```python
from build123d import *

# Parameters (mm, degrees)
SKETCH1_W           = 82.8
SKETCH1_H           = 57.7
BOSS_EXTRUDE1_DEPTH = 21.2
SKETCH2_R           = 1.5
CUT_EXTRUDE1_DEPTH  = 22
CUT_EXTRUDE2_DEPTH  = 20
FILLET3_R           = 4
BOSS_EXTRUDE3_START = 1
BOSS_EXTRUDE3_DEPTH = 1
CUT_EXTRUDE6_DEPTH  = 126.949440358
SKETCH8_R           = 3.8
CUT_EXTRUDE7_DEPTH  = 91.96532852
CUT_EXTRUDE8_DEPTH  = 10


with BuildPart() as part:
    # Sketch1 → Boss-Extrude1 (new body)
    with BuildSketch(Plane(origin=(0, 0, 0), x_dir=(1, 0, 0), z_dir=(0, 1, 0))):
        with Locations((-68.529666271, 2.285365627)):
            Rectangle(SKETCH1_W, SKETCH1_H)
    extrude(amount=BOSS_EXTRUDE1_DEPTH)

    # Sketch2 → Cut-Extrude1 (cut)
    with BuildSketch(Plane.XZ):
        with Locations(Location((-105.929666271, 22.574078856, 0), (0, 0, 270))):
            Circle(SKETCH2_R)
        with Locations(Location((-31.129666271, 22.574078856, 0), (0, 0, 270))):
            Circle(SKETCH2_R)
        with Locations(Location((-105.929666271, -27.14481011, 0), (0, 0, 270))):
            Circle(SKETCH2_R)
        with Locations(Location((-31.129666271, -27.14481011, 0), (0, 0, 270))):
            Circle(SKETCH2_R)
    extrude(amount=-CUT_EXTRUDE1_DEPTH, mode=Mode.SUBTRACT)

    # Sketch3 → Cut-Extrude2 (cut)
    with BuildSketch(Plane.XZ):
        with BuildLine():
            Line((-101.969305307, 23.064634373), (-35.090027235, 23.064634373))
            ThreePointArc((-35.090027235, 23.064634373), (-33.948648913, 19.745651731), (-30.629666271, 18.604273409))
            Line((-30.629666271, 18.604273409), (-30.629666271, -23.175004663))
            ThreePointArc((-30.629666271, -23.175004663), (-33.948648913, -24.316382985), (-35.090027235, -27.635365627))
            Line((-35.090027235, -27.635365627), (-101.969305307, -27.635365627))
            ThreePointArc((-101.969305307, -27.635365627), (-103.110683629, -24.316382985), (-106.429666271, -23.175004663))
            Line((-106.429666271, -23.175004663), (-106.429666271, 18.607164142))
            ThreePointArc((-106.429666271, 18.607164142), (-103.111962249, 19.747670443), (-101.969305307, 23.064634373))
        make_face()
    extrude(amount=-CUT_EXTRUDE2_DEPTH, mode=Mode.SUBTRACT)

    # Fillet3
    fillet3_edges = [part.edges().sort_by_distance(p)[0] for p in [
        (-27.129666271, 10.6, 26.564634373),
        (-109.929666271, 10.6, 26.564634373),
        (-109.929666271, 10.6, -31.135365627),
        (-27.129666271, 10.6, -31.135365627),
    ]]
    fillet(fillet3_edges, radius=FILLET3_R)

    # Sketch3_8 → Boss-Extrude3 (add)
    with BuildSketch(Plane.XZ.offset(BOSS_EXTRUDE3_START)):
        with BuildLine():
            Line((-103.334287863, 24.064634373), (-33.723727934, 24.064634373))
            ThreePointArc((-33.723727934, 24.064634373), (-33.241542132, 20.452758513), (-29.629666271, 19.97057271))
            Line((-29.629666271, 19.97057271), (-29.629666271, -24.541303964))
            ThreePointArc((-29.629666271, -24.541303964), (-33.241542132, -25.023489766), (-33.723727934, -28.635365627))
            Line((-33.723727934, -28.635365627), (-103.335604608, -28.635365627))
            ThreePointArc((-103.335604608, -28.635365627), (-103.817790411, -25.023489766), (-107.429666271, -24.541303964))
            Line((-107.429666271, -24.541303964), (-107.429666271, 19.973301106))
            ThreePointArc((-107.429666271, 19.973301106), (-103.819200468, 20.454646008), (-103.334287863, 24.064634373))
        make_face()
        with BuildLine():
            Line((-101.969305307, 23.064634373), (-35.090027235, 23.064634373))
            ThreePointArc((-35.090027235, 23.064634373), (-33.948648913, 19.745651731), (-30.629666271, 18.604273409))
            Line((-30.629666271, 18.604273409), (-30.629666271, -23.175004663))
            ThreePointArc((-30.629666271, -23.175004663), (-33.948648913, -24.316382985), (-35.090027235, -27.635365627))
            Line((-35.090027235, -27.635365627), (-101.969305307, -27.635365627))
            ThreePointArc((-101.969305307, -27.635365627), (-103.110683629, -24.316382985), (-106.429666271, -23.175004663))
            Line((-106.429666271, -23.175004663), (-106.429666271, 18.607164142))
            ThreePointArc((-106.429666271, 18.607164142), (-103.111962249, 19.747670443), (-101.969305307, 23.064634373))
        make_face(mode=Mode.SUBTRACT)
    extrude(amount=-BOSS_EXTRUDE3_DEPTH)

    # Sketch7 → Cut-Extrude6 (cut, through all)
    with BuildSketch(Plane(origin=(0, 0, -31.135365627), x_dir=(-1, 0, 0), z_dir=(0, 0, -1))):
        with BuildLine():
            Line((97.929666271, 10), (60.929666271, 10))
            ThreePointArc((60.929666271, 10), (59.929666271, 9), (60.929666271, 8))
            Line((60.929666271, 8), (97.929666271, 8))
            ThreePointArc((97.929666271, 8), (98.929666271, 9), (97.929666271, 10))
        make_face()
        with BuildLine():
            Line((97.929666271, 5), (60.929666271, 5))
            ThreePointArc((60.929666271, 5), (59.929666271, 4), (60.929666271, 3))
            Line((60.929666271, 3), (97.929666271, 3))
            ThreePointArc((97.929666271, 3), (98.929666271, 4), (97.929666271, 5))
        make_face()
    extrude(amount=-CUT_EXTRUDE6_DEPTH, mode=Mode.SUBTRACT)

    # Sketch8 → Cut-Extrude7 (cut, through all)
    with BuildSketch(Plane.ZY.offset(109.929666271)):
        with Locations((14.564634373, 9.2)):
            Circle(SKETCH8_R)
    extrude(amount=-CUT_EXTRUDE7_DEPTH, mode=Mode.SUBTRACT)

    # Sketch10 → Cut-Extrude8 (cut)
    with BuildSketch(Plane.XY.offset(26.564634373)):
        with BuildLine():
            Line((-43.129666271, 15), (-45.129666271, 15))
            ThreePointArc((-45.129666271, 15), (-47.129666271, 17), (-45.129666271, 19))
            Line((-45.129666271, 19), (-43.129666271, 19))
            ThreePointArc((-43.129666271, 19), (-41.129666271, 17), (-43.129666271, 15))
        make_face()
        with BuildLine():
            Line((-54.879666271, 15), (-56.879666271, 15))
            ThreePointArc((-56.879666271, 15), (-58.879666271, 17), (-56.879666271, 19))
            Line((-56.879666271, 19), (-54.879666271, 19))
            ThreePointArc((-54.879666271, 19), (-52.879666271, 17), (-54.879666271, 15))
        make_face()
        with BuildLine():
            Line((-66.629666271, 15), (-68.629666271, 15))
            ThreePointArc((-68.629666271, 15), (-70.629666271, 17), (-68.629666271, 19))
            Line((-68.629666271, 19), (-66.629666271, 19))
            ThreePointArc((-66.629666271, 19), (-64.629666271, 17), (-66.629666271, 15))
        make_face()
        with BuildLine():
            Line((-78.379666271, 15), (-80.379666271, 15))
            ThreePointArc((-80.379666271, 15), (-82.379666271, 17), (-80.379666271, 19))
            Line((-80.379666271, 19), (-78.379666271, 19))
            ThreePointArc((-78.379666271, 19), (-76.379666271, 17), (-78.379666271, 15))
        make_face()
    extrude(amount=-CUT_EXTRUDE8_DEPTH, mode=Mode.SUBTRACT)


solid = part.part
```
Can you work these out from the model? Positions are in its coordinate system, mm. A direction names the side the tool comes from. Round coordinates to 2 decimals unless told otherwise and drop trailing zeros. Loops run counter-clockwise (first coordinate to the right, second up) from the corner with the lowest first, then second, coordinate; pieces in that order, holes last.
Item 1: If we mould it in two halves opening along Z, with no side actions, what happens to faces 1 (the cylindrical face through (-33.91, 9.35, -24.28)), 2 (the cylindrical face through (-98.93, 3.98, 24.79)), 3 (the cylindrical face through (-28.33, 10.75, -29.99))? For each: +Z half, -Z half, draft (parallel to the pull), parting line (faces both ways), or undercut.
Item 2: Suppose I cut it at C-C, the plane y = 11.5. Write out the boundary of the cut face in (x, z) (3 decimals).
Item 3: Suppose I cut it at A-A, the plane y = 4. Write out the boundary of the cut face in (x, z) (3 decimals).
Item 4: Will these pins go through, and if not, where does the flat tip stop? pin 1 Ø3 at (x, z) = (-86.5, -29) entering from -Y; pin 2 Ø0.5 at (y, z) = (-0.5, 7.5) entering from -X; pin 3 Ø10 at (x, z) = (-77, 5) entering from -Y; pin 4 Ø1.8 at (x, z) = (-76, 25) entering from -Y.
Item 5: Please list where these lines run through material, in increasing order: L1, parallel to Y at x = -81.5, z = -28; L2, parallel to X at y = 17, z = 13.5; L3, parallel to Z at x = -105, y = 16.
Item 6: Suppose I cut it at D-D, the plane y = 17. State how many separate pieces and enclosed holes the cut face has, then the cut area to 3 significant figures.
Item 7: Suppose I cut it at B-B, the plane z = -11.5. Write out the boundary of the cut face in (x, y).
Item 8: Which directions (+Z, -Z, +X, -X, +Y, -Y) give clear straight access to the entire face, cutting with the end or side of a thin tool? Please do faces 4 (the cylindrical face through (-58.88, 16.96, 24.84)), 5 (the flat face through (-68, 12, -27.635)), 6 (the flat face through (-69, 21.2, -3)), 7 (the cylindrical face through (-28.904, 6.888, 11.549)), 8 (the flat face through (-79, 3, -29)).
Reported:
1. face 1: undercut
1. face 2: draft
1. face 3: -Z half
2. outline: (-109.93, -27.135) arc R4 ccw to (-105.93, -31.135) - (-31.13, -31.135) arc R4 ccw to (-27.13, -27.135) - (-27.13, 11.54) - (-30.63, 11.54) - (-30.63, -23.175) arc R4 ccw to (-35.09, -27.635) - (-101.969, -27.635) arc R4 ccw to (-106.43, -23.175) - (-106.43, 11.54) - (-109.93, 11.54) - close; (-109.93, 17.59) - (-106.43, 17.59) - (-106.43, 18.607) arc R4 ccw to (-101.969, 23.065) - (-35.09, 23.065) arc R4 ccw to (-30.63, 18.604) - (-30.63, 17.59) - (-27.13, 17.59) - (-27.13, 22.565) arc R4 ccw to (-31.13, 26.565) - (-105.93, 26.565) arc R4 ccw to (-109.93, 22.565) - close; hole circle Ø3 at (-105.93, -27.145); hole circle Ø3 at (-105.93, 22.574); hole circle Ø3 at (-31.13, -27.145); hole circle Ø3 at (-31.13, 22.574)
3. outline: (-109.93, -27.135) arc R4 ccw to (-105.93, -31.135) - (-98.93, -31.135) - (-98.93, -27.635) - (-101.969, -27.635) arc R4 ccw to (-106.43, -23.175) - (-106.43, 18.607) arc R4 ccw to (-101.969, 23.065) - (-98.93, 23.065) - (-98.93, 26.565) - (-105.93, 26.565) arc R4 ccw to (-109.93, 22.565) - close; (-59.93, -31.135) - (-31.13, -31.135) arc R4 ccw to (-27.13, -27.135) - (-27.13, 22.565) arc R4 ccw to (-31.13, 26.565) - (-59.93, 26.565) - (-59.93, 23.065) - (-35.09, 23.065) arc R4 ccw to (-30.63, 18.604) - (-30.63, -23.175) arc R4 ccw to (-35.09, -27.635) - (-59.93, -27.635) - close; hole circle Ø3 at (-105.93, -27.145); hole circle Ø3 at (-105.93, 22.574); hole circle Ø3 at (-31.13, -27.145); hole circle Ø3 at (-31.13, 22.574)
4. pin 1: stops at y = -1
4. pin 2: stops at x = -107.43
4. pin 3: stops at y = 20
4. pin 4: stops at y = 0
5. L1: y = -1 to 3, 5 to 8, 10 to 21.2
5. L2: x = -109.93 to -106.43, -30.63 to -27.13
5. L3: z = -31.14 to -28.32, -25.97 to -23.26, 18.69 to 21.4, 23.75 to 26.56
6. separate pieces: 4
6. enclosed holes: 4
6. area: 875 mm2
7. outline: (-109.93, 0) - (-107.43, 0) - (-107.43, -1) - (-106.43, -1) - (-106.43, 20) - (-30.63, 20) - (-30.63, -1) - (-29.63, -1) - (-29.63, 0) - (-27.13, 0) - (-27.13, 21.2) - (-109.93, 21.2) - close
8. face 4: +Z
8. face 5: -Y
8. face 6: +Z, -Z, +X, -X, +Y
8. face 7: +X, -X
8. face 8: +Z, -Z
